from build123d import *

# Parameters (mm, degrees)
SKETCH_1_R          = 18
EXTRUDE_1_DEPTH     = 13
SKETCH_2_R          = 13.5
EXTRUDE_2_DEPTH     = 1.5
SKETCH_3_R          = 15
EXTRUDE_3_DEPTH     = 14.5
SKETCH_4_R          = 14
EXTRUDE_4_DEPTH     = 23
SKETCH_5_R          = 12
EXTRUDE_5_DEPTH     = 34
SKETCH_6_R          = 16
EXTRUDE_6_DEPTH     = 25
EXTRUDE_START       = 31
SKETCH_7_R          = 15
EXTRUDE_7_DEPTH     = 31
CUT_EXTRUDE_START   = 11
CUT_EXTRUDE_1_DEPTH = 31
CUT_EXTRUDE_START_2 = 8
CUT_EXTRUDE_2_DEPTH = 31


with BuildPart() as part:
    # 草图1 → 凸台-拉伸1 (new body)
    with BuildSketch(Plane(origin=(0, 0, 0), x_dir=(0, 0, -1), z_dir=(1, 0, 0))):
        with Locations(Location((0, 0, 0), (0, 0, 180))):
            Circle(SKETCH_1_R)
    extrude(amount=EXTRUDE_1_DEPTH)

    # 草图2 → 凸台-拉伸2 (add)
    with BuildSketch(Plane(origin=(13, 0, 0), x_dir=(0, 0, -1), z_dir=(1, 0, 0))):
        Circle(SKETCH_2_R)
    extrude(amount=EXTRUDE_2_DEPTH)

    # 草图3 → 凸台-拉伸3 (add)
    with BuildSketch(Plane(origin=(14.5, 0, 0), x_dir=(0, 0, -1), z_dir=(1, 0, 0))):
        with Locations(Location((0, 0, 0), (0, 0, 180))):
            Circle(SKETCH_3_R)
    extrude(amount=EXTRUDE_3_DEPTH)

    # 草图4 → 凸台-拉伸4 (add)
    with BuildSketch(Plane(origin=(29, 0, 0), x_dir=(0, 0, -1), z_dir=(1, 0, 0))):
        Circle(SKETCH_4_R)
    extrude(amount=EXTRUDE_4_DEPTH)

    # 草图5 → 凸台-拉伸5 (add)
    with BuildSketch(Plane(origin=(52, 0, 0), x_dir=(0, 0, -1), z_dir=(1, 0, 0))):
        Circle(SKETCH_5_R)
    extrude(amount=EXTRUDE_5_DEPTH)

    # 草图6 → 凸台-拉伸6 (add)
    with BuildSketch(Plane.ZY):
        with Locations(Location((0, 0, 0), (0, 0, 180))):
            Circle(SKETCH_6_R)
    extrude(amount=EXTRUDE_6_DEPTH)

    # 草图7 → 凸台-拉伸7 (add)
    with BuildSketch(Plane.ZY.offset(25).offset(EXTRUDE_START)):
        Circle(SKETCH_7_R)
    extrude(amount=-EXTRUDE_7_DEPTH)

    # 草图8 → 切除-拉伸1 (cut)
    with BuildSketch(Plane.XY.offset(CUT_EXTRUDE_START)):
        with BuildLine():
            Line((-19, -5), (-7, -5))
            ThreePointArc((-7, -5), (-2, 0), (-7, 5))
            Line((-7, 5), (-19, 5))
            ThreePointArc((-19, 5), (-24, 0), (-19, -5))
        make_face()
    extrude(amount=CUT_EXTRUDE_1_DEPTH, mode=Mode.SUBTRACT)

    # 草图9 → 切除-拉伸2 (cut)
    with BuildSketch(Plane.XY.offset(CUT_EXTRUDE_START_2)):
        with BuildLine():
            Line((59, -4), (76, -4))
            ThreePointArc((76, -4), (80, 0), (76, 4))
            Line((76, 4), (59, 4))
            ThreePointArc((59, 4), (55, 0), (59, -4))
        make_face()
    extrude(amount=CUT_EXTRUDE_2_DEPTH, mode=Mode.SUBTRACT)


solid = part.part
Verification items for the finished model (mm, model axes). A direction names the side the tool comes from. Give positions to 0.01 mm unless a question says otherwise; leave off trailing zeros. Write each loop counter-clockwise with the first axis right and the second up, starting at its lowest first coordinate (ties: lowest second). Pieces come first, ordered by that corner, then holes. Notation, with made-up numbers: M 64,-19 L 76,-19 A24 cw 76,13 Z; hole C -10.5,82.5 d9. An arc over 180 degrees is marked long. Use CSV: the item, a comma, the result in double quotes.
1) Cross-section at C-C (y = -9). Enter the section's corners in (x, z), plus the area to 3 significant figures.
Final values:
outline,"M -56,-12 L -25,-12 L -25,-13.23 L 0,-13.23 L 0,-15.59 L 13,-15.59 L 13,-10.06 L 14.5,-10.06 L 14.5,-12 L 29,-12 L 29,-10.72 L 52,-10.72 L 52,-7.94 L 86,-7.94 L 86,7.94 L 52,7.94 L 52,10.72 L 29,10.72 L 29,12 L 14.5,12 L 14.5,10.06 L 13,10.06 L 13,15.59 L 0,15.59 L 0,13.23 L -25,13.23 L -25,12 L -56,12 Z"
area,"3,220 mm²"
2) Release check for a two-part mould opening along Y. For faces 1 (the face through (21.65, -12.65, 8.06)), 2 (the face through (-2, 0, 13)), 3 (the face through (-56, 0, 0)) record: released by +Y, released by -Y, zero draft, split by the parting line, or undercut.
Final values:
face 1,"split by the parting line"
face 2,"undercut"
face 3,"zero draft"
3) Cross-section at B-B (x = 43.5). Enter the section's corners in (y, z).
Final values:
outline,"C 0,0 d28"
4) Cross-section at A-A (z = 0). Enter the section's corners in (x, y).
Final values:
outline,"M -56,-15 L -25,-15 L -25,-16 L 0,-16 L 0,-18 L 13,-18 L 13,-13.5 L 14.5,-13.5 L 14.5,-15 L 29,-15 L 29,-14 L 52,-14 L 52,-12 L 86,-12 L 86,12 L 52,12 L 52,14 L 29,14 L 29,15 L 14.5,15 L 14.5,13.5 L 13,13.5 L 13,18 L 0,18 L 0,16 L -25,16 L -25,15 L -56,15 Z"
5) Access from +Z, -Z, +X, -X, +Y, -Y to the whole of each face (thin tool, end or side, straight path). Record for faces 4 (the face through (14.5, -7.85, -11.18)), 5 (the face through (0, 11, -12)), 6 (the face through (-24, 0, 13)), 7 (the face through (68.762, -4.596, -11.085)).
Final values:
face 4,"none"
face 5,"-X"
face 6,"+Z"
face 7,"+X"
6) Cross-section at D-D (x = -34). Enter the section's corners in (y, z).
Final values:
outline,"C 0,0 d30"
7) Material ranges on line 1 along X through (y, z) = (6, -13); line 2 along X through (y, z) = (-12, -13); line 3 along Y through (x, z) = (59, -5), recorded low to high.
Final values:
line 1,"-56 to 13, 14.5 to 29"
line 2,"0 to 13"
line 3,"-10.91 to 10.91"
8) Go/stop test with flat-tipped pins: pin 1 Ø10 at (x, z) = (-22.5, 3) entering from -Y; pin 2 Ø5 at (x, z) = (-20, -5.5) entering from -Y; pin 3 Ø6.5 at (x, y) = (72, 0) entering from +Z. Record where each tip stops, or that it passes through.
Final values:
pin 1,"y = -16"
pin 2,"y = -15.72"
pin 3,"z = 8"
